Read the model definition and answer for the solid it produces. Units are mm, in the model's axes. A direction names the side the tool comes from. Coordinates: 2 decimals unless noted, no trailing zeros. Write each loop counter-clockwise with the first axis right and the second up, starting at its lowest first coordinate (ties: lowest second). Pieces come first, ordered by that corner, then holes. Notation, with made-up numbers: (3, -26.5) -> (33, -26.5) arc R13 ccw to (33, -20.5) -> close; hole circle Ø1 at (-1.5, -13). An arc over 180 degrees is marked (long way). Write item = value, one per line. Start each with the question number.
1) Section C-C (z = -5.5) is taken. Determine the outline of the cut face in (x, y) (1 decimal).
2) Section D-D (x = -1.9) is taken. Determine the outline of the cut face in (y, z).
3) Section A-A (y = 0) is taken. Determine the outline of the cut face in (x, z).
4) Flat-ended cylindrical pins translate along their axes: pin 1 Ø1.2 at (x, z) = (-1, 1.5) entering from +Y; pin 2 Ø1.5 at (y, z) = (-1.5, -2) entering from +X; pin 3 Ø0.6 at (y, z) = (1, 1.5) entering from +X. Find the tip coordinate at first contact, or state that the pin passes through.
5) A tool of negligible diameter and unlimited length cuts with its end or side. For faces 4 (the face through (2.569, 1.065, 0.334)), 5 (the face through (2, 0, 0)), 6 (the face through (-0.404, -1, 1)), from which of +Z, -Z, +X, -X, +Y, -Y can it reach the whole face along a straight path? Write none if from no direction.
6) For a pull along Y with two mould halves and no side action, classify faces 1 (the face through (-0.34, 1.55, -6.25)), 2 (the face through (0, 0, -12.7)), 3 (the face through (1, -0.404, 1)) as released by +Y, released by -Y, zero draft, split by the parting line, or undercut.
7) Find the intervals of material crossed by line 1 along X through (y, z) = (-0.1, -8.5); line 2 along Y through (x, z) = (-0.25, -0.5); line 3 along Z through (x, y) = (-2.2, -1.6), in increasing order. Write a range as from..to.
Solid Edge part; units mm, degrees
sketch "Sketch1" plane through (0, 0, 0) normal (0, -1, 0) x (1, 0, 0)
  arc A0 (0, 2.032) -> (2.7813, 0.6773) centre (0, -1.5005) cw
  line L0 (2.7813, 0.6773) -> (2.7813, 0)
  line L1 (2.7813, 0) -> (1.5875, 0)
  line L2 (1.5875, 0) -> (1.5875, -12.3334)
  line L3 (1.5875, -12.3334) -> (0.9525, -12.7)
  line L4 (0.9525, -12.7) -> (0, -12.7)
  dimension "D1" = 2.7813
  dimension "D2" = 2.7813
  dimension "D3" = 2.7813
revolve "RevolvedProtrusion1" add sketch "Sketch1" angle 360 about axis through (0, 0, 0) along (0, 0, 1)
sketch "Sketch2" plane through (0, 0, 0.6773) normal (0, 0, 1) x (1, 0, 0)
  line L0 (0.4041, -0.4041) -> (1.5352, -0.4041)
  line L1 (1.5352, -0.4041) -> (1.5352, 0.4041)
  line L2 (1.5352, 0.4041) -> (0.4041, 0.4041)
  line L3 (0.4041, 0.4041) -> (0.4041, 1.5352)
  line L4 (0.4041, 1.5352) -> (-0.4041, 1.5352)
  line L5 (-0.4041, 1.5352) -> (-0.4041, 0.4041)
  line L6 (-0.4041, 0.4041) -> (-1.5352, 0.4041)
  line L7 (-1.5352, 0.4041) -> (-1.5352, -0.4041)
  line L8 (-1.5352, -0.4041) -> (-0.4041, -0.4041)
  line L9 (-0.4041, -0.4041) -> (-0.4041, -1.5352)
  line L10 (-0.4041, -1.5352) -> (0.4041, -1.5352)
  line L11 (0.4041, -1.5352) -> (0.4041, -0.4041)
extrude "Cutout1" cut sketch "Sketch2" along normal through all
cosmetic_thread "Thread1"
properties material "Acier galvanisé"
Answer key:
q1.outline = circle Ø3.2 at (0, 0)
q2.outline = (-2.03, 0) -> (2.03, 0) -> (2.03, 0.68) arc R2.98 ccw to (-2.03, 0.68) -> close
q3.outline = (-2.78, 0) -> (-1.59, 0) -> (-1.59, -12.33) -> (-0.95, -12.7) -> (0.95, -12.7) -> (1.59, -12.33) -> (1.59, 0) -> (2.78, 0) -> (2.78, 0.68) arc R3.53 ccw to (1.54, 1.68) -> (1.54, 0.68) -> (-1.54, 0.68) -> (-1.54, 1.68) arc R3.53 ccw to (-2.78, 0.68) -> close
q4.pin_1 = 2.43
q4.pin_2 = 1.4
q4.pin_3 = 2.07
q5.face_4 = +Z, -Z
q5.face_5 = -Z
q5.face_6 = +Z
q6.face_1 = split by the parting line
q6.face_2 = zero draft
q6.face_3 = undercut
q7.line_1 = -1.58..1.58
q7.line_2 = -1.57..1.57
q7.line_3 = 0..0.75
